Could you check a few things on this model? Use its own coordinates, in mm. Coordinates: 2 decimals unless noted, no trailing zeros. Order: outer loops, then holes, each group sorted by start corner. A loop starts at its lowest first (then second) coordinate and runs counter-clockwise, first axis right, second up. Notation, with made-up numbers: (34.5, 45.25) - (85.5, 45.25) arc R34 cw to (85.5, 80.25) - close; hole circle Ø10 at (-8, -11). An arc over 180 degrees is marked (long way). Answer as a JSON object with one key per item and string values. Group by question number.
(1) Imagine slicing it at A-A, the plane z = 6. Write out the boundary of the cut face in (x, y), and give its area (3 significant figures).
(2) Will these pins go through, and if not, where does the flat tip stop? P1, Ø5, axis at y = 2.5, z = 7, coming from the -X side; P2, Ø6, axis at x = 18.5, y = 5, coming from the -Z side; P3, Ø0.5, axis at x = 31, y = 0, coming from the +Z side.
(3) We'd pull the mould along X, two halves only. Please class faces 1 (the flat face through (-1, 0, 0)), 2 (the cylindrical face through (29.6, 0.07, 1.73)), 3 (the flat face through (-10, 0, 10)): pulls with the +X half, pulls with the -X half, needs draft (parallel to the pull), parting line crosses it, or undercut.
(4) Please list where these lines run through material, in increasing order: probe 1 along X at (y, z) = (2, 6); probe 2 along X at (y, z) = (1.75, 1.25); probe 3 along Z at (x, y) = (15.5, -3.5).
from build123d import *

# Parameters (mm, degrees)
F2_ANGLE = 180
F3_R     = 1.5
F4_DEPTH = 4.5
F3_R_2   = 2.5
F5_DEPTH = 10
F6_SIZE  = 1


with BuildPart() as f2:
    # F1 (on Top) → F2 (revolve)
    with BuildSketch(Plane.XY):
        with BuildLine():
            Line((45, 0), (-45, 0))
            add(Edge.make_bspline(
                [(-45, 0), (-45, -5.698118126), (-19.5767879486, -5.9), (0, -6.1)],
                knots=[0, 0, 0, 0, 1, 1, 1, 1], degree=3))
            add(Edge.make_bspline(
                [(45, 0), (45, -5.698118126), (19.5767879486, -5.9), (0, -6.1)],
                knots=[0, 0, 0, 0, 1, 1, 1, 1], degree=3))
        make_face()
    revolve(axis=Axis((0, 0, 0), (1, 0, 0)), revolution_arc=F2_ANGLE)

    # F3 (on face) → F4 (join)
    with BuildSketch(Plane.XY):
        with Locations((-30.5, 0)):
            Circle(F3_R)
        with Locations((31.1, 0)):
            Circle(F3_R)
    extrude(amount=F4_DEPTH)

    # F3 (on face) → F5 (join)
    with BuildSketch(Plane.XY):
        with Locations((-9.9, 0)):
            Circle(F3_R_2)
    extrude(amount=F5_DEPTH)

    # F6
    f6_edges = [f2.edges().sort_by_distance(p)[0] for p in [
        (-32, 0, 4.5),
        (-12.4, 0, 10),
        (29.6, 0, 4.5),
    ]]
    chamfer(f6_edges, length=F6_SIZE)


solid = f2.part
Result set:
{
 "1": {"outline": "circle Ø5 at (-9.9, 0)", "area": "19.6 mm^2"},
 "2": {"P1": "stops at x = -12.4", "P2": "stops at z = -5.41", "P3": "stops at z = 4.5"},
 "3": {"face 1": "undercut", "face 2": "undercut", "face 3": "needs draft"},
 "4": {"probe 1": "x = -11.4 to -8.4", "probe 2": "x = -11.69 to -8.11", "probe 3": "z = -4.7 to 0"}
}
